Model file for the job. Use its own axes, mm. A direction names the side the tool comes from. Give positions to 0.01 mm unless a question says otherwise; leave off trailing zeros. Write each loop counter-clockwise with the first axis right and the second up, starting at its lowest first coordinate (ties: lowest second). Pieces come first, ordered by that corner, then holes. Notation, with made-up numbers: (46, 72) - (75, 72) arc R12 ccw to (75, 91) - close; hole circle Ø11 at (65.25, -31). An arc over 180 degrees is marked (long way). One line per item, written item: value. Start each with the question number.
(1) Mould opens along X. For faces 3 (the face through (-7, 31, 79)), 4 (the face through (-1, 1, 85)), 5 (the face through (-33.727, -25.861, 41.905)) say: pulls with the +X half, pulls with the -X half, needs draft (parallel to the pull), parting line crosses it, or undercut.
(2) Probe L1, parallel to X at y = -25.5, z = 34.5; L2, parallel to Y at x = -15, z = 35.5; L3, parallel to Y at x = -16, z = 61. List the from-to ranges inside material, lowest first.
(3) 3-axis set-ups, long thin cutter, end or side, ignore diameter. For faces 1 (the face through (-5.458, 31.452, 82.042)), 2 (the face through (-23, -26, 42)): which of +Z, -Z, +X, -X, +Y, -Y reach the whole face in a straight line?
(4) Drop flat-ended pins along their axis: P1, Ø12, axis at x = -5, z = 73.5, coming from the +Y side; P2, Ø1.5, axis at x = 30.5, y = 9, coming from the +Z side; P3, Ø0.8, axis at y = 8.5, z = 82, coming from the +X side; P4, Ø9.5, axis at x = -15, y = 25.98, coming from the +Z side. Give the stop position or say it passes through.
(5) Cut at D-D, the plane z = 39. List the corners of the cut face in (x, y), and give its area (3 significant figures).
(6) Cut at B-B, the plane y = 6.5. List the corners of the cut face in (x, z), and give its area (3 significant figures).
(7) Cut at C-C, the plane x = 30. List the corners of the cut face in (y, z), and give its area (3 significant figures).
(8) Cut at A-A, the plane x = -13. List the corners of the cut face in (y, z).
from build123d import *

# Parameters (mm, degrees)
F0_R     = 42.5
F0_R_2   = 8
F1_DEPTH = 85
F3_DEPTH = 6


with BuildPart() as f1:
    # F0 (on Top) → F1 (new body)
    with BuildSketch(Plane.XY):
        Circle(F0_R)
        with Locations((-15, -25.9807621135)):
            Circle(F0_R_2, mode=Mode.SUBTRACT)
        with Locations((-15, 25.9807621135)):
            Circle(F0_R_2, mode=Mode.SUBTRACT)
        with Locations((30, 0)):
            Circle(F0_R_2, mode=Mode.SUBTRACT)
    extrude(amount=F1_DEPTH)

    # F2 (on face) → F3 (cut)
    with BuildSketch(Plane.XY.offset(85)):
        with BuildLine():
            ThreePointArc((28.5, 7.8581168228), (30, 8), (31.5, 7.8581168228))
            Line((31.5, 7.8581168228), (31.5, 9.5))
            ThreePointArc((31.5, 9.5), (30, 11), (28.5, 9.5))
            Line((28.5, 9.5), (28.5, 7.8581168228))
        make_face()
        with BuildLine():
            Line((31.5, -9.5), (31.5, -7.8581168228))
            ThreePointArc((31.5, -7.8581168228), (30, -8), (28.5, -7.8581168228))
            Line((28.5, -7.8581168228), (28.5, -9.5))
            ThreePointArc((28.5, -9.5), (30, -11), (31.5, -9.5))
        make_face()
        with BuildLine():
            Line((-8.9446712056, -31.2088586306), (-7.522758664, -32.0298002192))
            ThreePointArc((-7.522758664, -32.0298002192), (-5.4737205584, -31.4807621135), (-6.022758664, -29.4317240079))
            Line((-6.022758664, -29.4317240079), (-7.4446712056, -28.6107824192))
            ThreePointArc((-7.4446712056, -28.6107824192), (-8.0717967697, -29.9807621135), (-8.9446712056, -31.2088586306))
        make_face()
        with BuildLine():
            Line((-23.977241336, -22.5298002192), (-22.5553287944, -23.3507418078))
            ThreePointArc((-22.5553287944, -23.3507418078), (-21.9282032303, -21.9807621135), (-21.0553287944, -20.7526655965))
            Line((-21.0553287944, -20.7526655965), (-22.477241336, -19.9317240079))
            ThreePointArc((-22.477241336, -19.9317240079), (-24.5262794416, -20.4807621135), (-23.977241336, -22.5298002192))
        make_face()
        with BuildLine():
            Line((-22.5553287944, 23.3507418078), (-23.977241336, 22.5298002192))
            ThreePointArc((-23.977241336, 22.5298002192), (-24.5262794416, 20.4807621135), (-22.477241336, 19.9317240079))
            Line((-22.477241336, 19.9317240079), (-21.0553287944, 20.7526655965))
            ThreePointArc((-21.0553287944, 20.7526655965), (-21.9282032303, 21.9807621135), (-22.5553287944, 23.3507418078))
        make_face()
        with BuildLine():
            Line((-7.522758664, 32.0298002192), (-8.9446712056, 31.2088586306))
            ThreePointArc((-8.9446712056, 31.2088586306), (-8.0717967697, 29.9807621135), (-7.4446712056, 28.6107824192))
            Line((-7.4446712056, 28.6107824192), (-6.022758664, 29.4317240079))
            ThreePointArc((-6.022758664, 29.4317240079), (-5.4737205584, 31.4807621135), (-7.522758664, 32.0298002192))
        make_face()
    extrude(amount=-F3_DEPTH, mode=Mode.SUBTRACT)


solid = f1.part
Answers follow:
1. face 3: undercut
1. face 4: needs draft
1. face 5: parting line crosses it
2. L1: x = -34 to -22.99, -7.01 to 34
2. L2: y = -39.76 to -33.98, -17.98 to 17.98, 33.98 to 39.76
2. L3: y = -39.37 to -33.92, -18.04 to 18.04, 33.92 to 39.37
3. face 1: +Z
3. face 2: +Z, -Z
4. P1: stops at y = 42.5
4. P2: stops at z = 79
4. P3: stops at x = 41.72
4. P4: passes through
5. outline: circle Ø85 at (0, 0); hole circle Ø16 at (-15, -25.98); hole circle Ø16 at (-15, 25.98); hole circle Ø16 at (30, 0)
5. area: 5,070 mm²
6. outline: (-42, 0) - (25.34, 0) - (25.34, 85) - (-42, 85) - close; (34.66, 0) - (42, 0) - (42, 85) - (34.66, 85) - close
6. area: 6,350 mm²
7. outline: (-30.1, 0) - (-8, 0) - (-8, 79) - (-11, 79) - (-11, 85) - (-30.1, 85) - close; (8, 0) - (30.1, 0) - (30.1, 85) - (11, 85) - (11, 79) - (8, 79) - close
7. area: 3,720 mm²
8. outline: (-40.46, 0) - (-33.73, 0) - (-33.73, 85) - (-40.46, 85) - close; (-18.23, 0) - (18.23, 0) - (18.23, 85) - (-18.23, 85) - close; (33.73, 0) - (40.46, 0) - (40.46, 85) - (33.73, 85) - close
